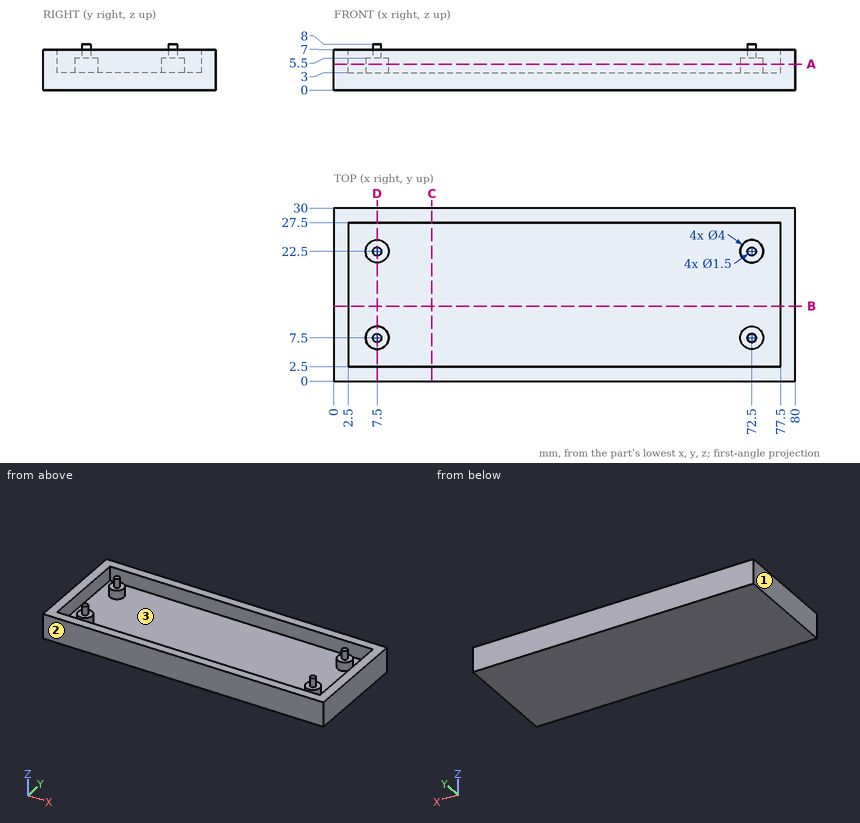
Input: dimensioned drawing with shaded views. Units: mm. Origin: part minimum x, y, z. Coordinates: 2 decimals unless noted, no trailing zeros. Loops run counter-clockwise (first coordinate to the right, second up) from the corner with the lowest first, then second, coordinate; pieces in that order, holes last. Notation, with made-up numbers: M -18,-22 L 35,-22 A25 cw 35,-6 Z; hole C -26.5,-34.75 d6. An arc over 180 degrees is marked long. Use a Markdown table: item, result. Add a question column.
1) Section A-A, the plane z = 4.5. Return the cut outline in (x, y), plus the area to 3 significant figures.
2) Line query: L1, parallel to Y at x = 5.5, z = 6.5; L2, parallel to X at y = 22.5, z = 3.5; L3, parallel to X at y = 20, z = 6.5. Output: solid intervals per line, ascending. Write a range as from..to.
3) Section C-C, the plane x = 17. Return the cut outline in (y, z).
4) Draft query along Y for the marked faces 1, 2 and 3. Return one class per face: +Y half, -Y half, draft (parallel to the pull), parting line (faces both ways), or undercut.
5) Section D-D, the plane x = 7.5. Return the cut outline in (y, z).
6) Section B-B, the plane y = 13. Return the cut outline in (x, z), plus the area to 3 significant figures.
7) Pin query (flat end, axial travel): P1, Ø3, axis at y = 16, z = 5.5, coming from the -X side; P2, Ø8, axis at x = 27, y = 11, coming from the +Z side. Return the tip coordinate at first contact, or that it passes through.
Answer below:
| question | item | result |
|---|---|---|
| 1 | outline | M 0,0 L 80,0 L 80,30 L 0,30 Z; C 7.5,7.5 d4; C 7.5,22.5 d4; C 72.5,7.5 d4; C 72.5,22.5 d4; hole M 2.5,2.5 L 77.5,2.5 L 77.5,27.5 L 2.5,27.5 Z |
| 1 | area | 575 mm2 |
| 2 | L1 | 0..2.5, 27.5..30 |
| 2 | L2 | 0..2.5, 5.5..9.5, 70.5..74.5, 77.5..80 |
| 2 | L3 | 0..2.5, 77.5..80 |
| 3 | outline | M 0,0 L 30,0 L 30,7 L 27.5,7 L 27.5,3 L 2.5,3 L 2.5,7 L 0,7 Z |
| 4 | face 1 | draft |
| 4 | face 2 | -Y half |
| 4 | face 3 | undercut |
| 5 | outline | M 0,0 L 30,0 L 30,7 L 27.5,7 L 27.5,3 L 24.5,3 L 24.5,5.5 L 23.25,5.5 L 23.25,8 L 21.75,8 L 21.75,5.5 L 20.5,5.5 L 20.5,3 L 9.5,3 L 9.5,5.5 L 8.25,5.5 L 8.25,8 L 6.75,8 L 6.75,5.5 L 5.5,5.5 L 5.5,3 L 2.5,3 L 2.5,7 L 0,7 Z |
| 6 | outline | M 0,0 L 80,0 L 80,7 L 77.5,7 L 77.5,3 L 2.5,3 L 2.5,7 L 0,7 Z |
| 6 | area | 260 mm2 |
| 7 | P1 | x = 0 |
| 7 | P2 | z = 3 |
